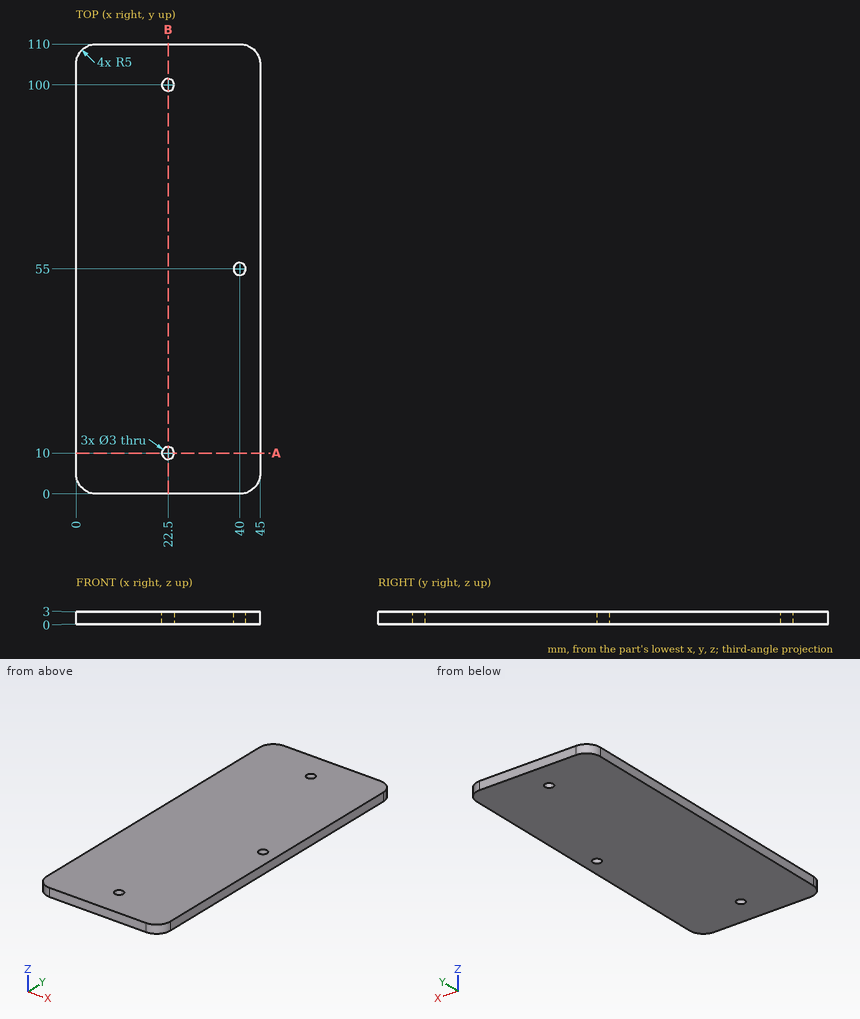
Answer from the drawing. Dimensions are ordinates in mm from the lowest x, y and z of the part. Round coordinates to 2 decimals unless told otherwise and drop trailing zeros. Write each loop counter-clockwise with the first axis right and the second up, starting at its lowest first coordinate (ties: lowest second). Pieces come first, ordered by that corner, then holes. Notation, with made-up numbers: (84.5, 34) - (97.5, 34) arc R17 ccw to (97.5, 48) - close; hole circle Ø5 at (13.5, -8). An arc over 180 degrees is marked (long way). Use a Markdown table: item, result.
(1) The part is cut by section A-A (y = 10). Write down the section's boundary in (x, z).
Reported:
| item | result |
|---|---|
| outline | (0, 0) - (21, 0) - (21, 3) - (0, 3) - close; (24, 0) - (45, 0) - (45, 3) - (24, 3) - close |
(2) This flat-tipped pin is pushed along its axis until it touches: pin 1 Ø2.5 at (x, y) = (22.5, 100) entering from +Z. Where does it stop, or does it pass through?
Reported:
| item | result |
|---|---|
| pin 1 | through |
(3) Straight lines are drawn through the part: line 1 along Y through (x, z) = (22.5, 2.45); line 2 along X through (y, z) = (100, 1.9); line 3 along Y through (x, z) = (39, 1.55). For each, find the intervals that lie inside material, in ascending order. Write a range as [from, to].
Reported:
| item | result |
|---|---|
| line 1 | [0, 8.5], [11.5, 98.5], [101.5, 110] |
| line 2 | [0, 21], [24, 45] |
| line 3 | [0, 53.88], [56.12, 110] |
(4) The part is cut by section B-B (x = 22.5). Write down the section's boundary in (y, z).
Reported:
| item | result |
|---|---|
| outline | (0, 0) - (8.5, 0) - (8.5, 3) - (0, 3) - close; (11.5, 0) - (98.5, 0) - (98.5, 3) - (11.5, 3) - close; (101.5, 0) - (110, 0) - (110, 3) - (101.5, 3) - close |
